Autodesk Inventor part; units mm, degrees
ref_plane "YZ Plane" through (0, 0, 0) normal (1, 0, 0) x (0, 1, 0)
ref_plane "XZ Plane" through (0, 0, 0) normal (0, 1, 0) x (-1, 0, 0)
ref_plane "XY Plane" through (0, 0, 0) normal (0, 0, 1) x (1, 0, 0)
sketch "Sketch1" plane through (0, 0, 0) normal (0, 0, 1) x (1, 0, 0)
  line L0 (52.5, 200) -> (-52.5, 200)
  line L1 (-52.5, 200) -> (-52.5, 0)
  line L2 (-52.5, 0) -> (52.5, 0)
  line L3 (52.5, 0) -> (52.5, 200)
  point P0 (0, 0)
  point P1 (0, 0)
  dimension "d0" = 105
  dimension "d1" = 200
extrude "Extrusion1" add sketch "Sketch1" along normal mid plane 80
fillet "Fillet1" radius 12 8 edges at (52.5, 100, 40) (52.5, 100, -40) (-52.5, 100, 40) (-52.5, 100, -40) (0, 0, 40) (-52.5, 0, 0) (0, 0, -40) (52.5, 0, 0)
shell "Shell1" thickness 2 removed faces 1 at (-13.5, 200, 13.3333)
sketch "Sketch2" plane through (-40.5, 0, 28) normal (0, -1, 0) x (1, 0, 0)
  circle A0 centre (40.5, -28) radius 25 construction
  circle A1 centre (40.5, -28) radius 23
  dimension "d6" = 2
  dimension "d9" = 50
extrude "Extrusion2" cut sketch "Sketch2" against normal blind 5
properties part number "silo"
Verification items for the finished model (mm, model axes). A direction names the side the tool comes from. Coordinates: 2 decimals unless noted, no trailing zeros. Order: outer loops, then holes, each group sorted by start corner. A loop starts at its lowest first (then second) coordinate and runs counter-clockwise, first axis right, second up. Notation, with made-up numbers: (-17, -27) -> (7, -27) arc R26 cw to (7, -11) -> close; hole circle Ø1 at (15, 54). An arc over 180 degrees is marked (long way). Answer as CSV lines item,"result". Start each with the question number.
1) Cross-section at D-D, the plane x = -31.5. Record the boundary of the cut face in (y, z), then the cut area to 3 significant figures.
2) Gauge pin test, flat ends, axial feed: pin 1 Ø10 at (x, z) = (12.5, -25.5) entering from +Y; pin 2 Ø17 at (x, z) = (13, 8) entering from +Y. Record the tip position at first contact, or that the pin passes through.
3) Material ranges on L1, parallel to X at y = 33.5, z = -26.5; L2, parallel to Z at x = 33.5, y = 130.5; L3, parallel to Y at x = 38, z = -12, recorded low to high. Write a range as [from, to].
4) Cross-section at B-B, the plane x = 0. Record the boundary of the cut face in (y, z), then the cut area to 3 significant figures.
5) Cross-section at A-A, the plane z = 0. Record the boundary of the cut face in (x, y).
6) Cross-section at C-C, the plane y = 110.5. Record the boundary of the cut face in (x, z).
7) Set-up check for faces 4 (the face through (-2.994, 0.986, 22.804)), 5 (the face through (-47.49, 104.68, 35.15)): record each of +Z, -Z, +X, -X, +Y, -Y from which the full face is reachable in a straight line by a thin tool's end or side.
8) Release check for a two-part mould opening along Z. For faces 1 (the face through (52.5, 105, 0)), 2 (the face through (-50.5, 107, 0)), 3 (the face through (-48.89, 104.68, 36.58)) record: released by +Z, released by -Z, zero draft, split by the parting line, or undercut.
Conclusion:
1,outline,"(0, -28) arc R12 ccw to (12, -40) -> (200, -40) -> (200, -38) -> (12, -38) arc R10 cw to (2, -28) -> (2, 28) arc R10 cw to (12, 38) -> (200, 38) -> (200, 40) -> (12, 40) arc R12 ccw to (0, 28) -> close"
1,area,"933 mm²"
2,pin 1,"stops at y = 2.32"
2,pin 2,"stops at y = 2"
3,L1,"x = [-52.5, -50.5], [50.5, 52.5]"
3,L2,"z = [-40, -38], [38, 40]"
3,L3,"y = [0, 2]"
4,outline,"(0, -28) arc R12 ccw to (12, -40) -> (200, -40) -> (200, -38) -> (12, -38) arc R10 cw to (2, -28) -> (2, -23) -> (0, -23) -> close; (0, 23) -> (2, 23) -> (2, 28) arc R10 cw to (12, 38) -> (200, 38) -> (200, 40) -> (12, 40) arc R12 ccw to (0, 28) -> close"
4,area,"841 mm²"
5,outline,"(-52.5, 12) arc R12 ccw to (-40.5, 0) -> (-23, 0) -> (-23, 2) -> (-40.5, 2) arc R10 cw to (-50.5, 12) -> (-50.5, 200) -> (-52.5, 200) -> close; (23, 0) -> (40.5, 0) arc R12 ccw to (52.5, 12) -> (52.5, 200) -> (50.5, 200) -> (50.5, 12) arc R10 cw to (40.5, 2) -> (23, 2) -> close"
6,outline,"(-52.5, -28) arc R12 ccw to (-40.5, -40) -> (40.5, -40) arc R12 ccw to (52.5, -28) -> (52.5, 28) arc R12 ccw to (40.5, 40) -> (-40.5, 40) arc R12 ccw to (-52.5, 28) -> close; hole (-50.5, -28) arc R10 ccw to (-40.5, -38) -> (40.5, -38) arc R10 ccw to (50.5, -28) -> (50.5, 28) arc R10 ccw to (40.5, 38) -> (-40.5, 38) arc R10 ccw to (-50.5, 28) -> close"
7,face 4,"+Y, -Y"
7,face 5,"+Y"
8,face 1,"zero draft"
8,face 2,"undercut"
8,face 3,"released by +Z"
